```python
from build123d import *

# Parameters (mm, degrees)
SKETCH1_R           = 3.5
BOSS_EXTRUDE1_DEPTH = 100
SKETCH2_R           = 5
BOSS_EXTRUDE2_DEPTH = 4
FILLET3_R           = 4


with BuildPart() as part:
    # Sketch1 → Boss-Extrude1 (new body)
    with BuildSketch(Plane(origin=(0, 0, 0), x_dir=(1, 0, 0), z_dir=(0, 1, 0))):
        with Locations(Location((0, 0, 0), (0, 0, 270))):
            Circle(SKETCH1_R)
    extrude(amount=-BOSS_EXTRUDE1_DEPTH)

    # Sketch2 → Boss-Extrude2 (add)
    with BuildSketch(Plane(origin=(0, 0, 0), x_dir=(1, 0, 0), z_dir=(0, 1, 0))):
        with Locations(Location((0, 0, 0), (0, 0, 270))):
            Circle(SKETCH2_R)
    extrude(amount=BOSS_EXTRUDE2_DEPTH)

    # Fillet3
    fillet3_edges = [part.edges().sort_by_distance(p)[0] for p in [
        (0, 4, -5),
    ]]
    fillet(fillet3_edges, radius=FILLET3_R - 0.0001)  # a hair under: the kernel refuses the full size


solid = part.part
```
The listing builds one solid part. Answer for the finished solid, in the listing's coordinates (mm). A direction names the side the tool comes from. Give positions to 0.01 mm unless a question says otherwise; leave off trailing zeros. Order: outer loops, then holes, each group sorted by start corner. A loop starts at its lowest first (then second) coordinate and runs counter-clockwise, first axis right, second up.
Item 1: The part is cut by section A-A, the plane y = -72.5. Give the vertices of the cut face in (x, z).
From the geometry:
outline: circle Ø7 at (0, 0)
Item 2: Given pin 1 Ø1.5 at (x, y) = (3.5, -65) entering from +Z; pin 2 Ø4 at (y, z) = (-55.5, 0.5) entering from -X; pin 3 Ø6 at (y, z) = (-24, -0.5) entering from +X, each flat-ended and moving along its own axis, determine where each tip first touches the part or whether it passes through.
From the geometry:
pin 1: stops at z = 2.17
pin 2: stops at x = -3.5
pin 3: stops at x = 3.5
Item 3: Find the intervals of material crossed by probe 1 along Y at (x, z) = (-0.5, 1); probe 2 along Z at (x, y) = (-0.25, -17.5), in increasing order.
From the geometry:
probe 1: y = -100 to 4
probe 2: z = -3.49 to 3.49
Item 4: Which of the six approach directions +Z, -Z, +X, -X, +Y, -Y give full straight-line access (tool end or side, diameter ignored) to faces 1 (the face through (0, 4, 0)), 2 (the face through (-3.3, 0, 2.2))?
From the geometry:
face 1: +Z, -Z, +X, -X, +Y
face 2: -Y
